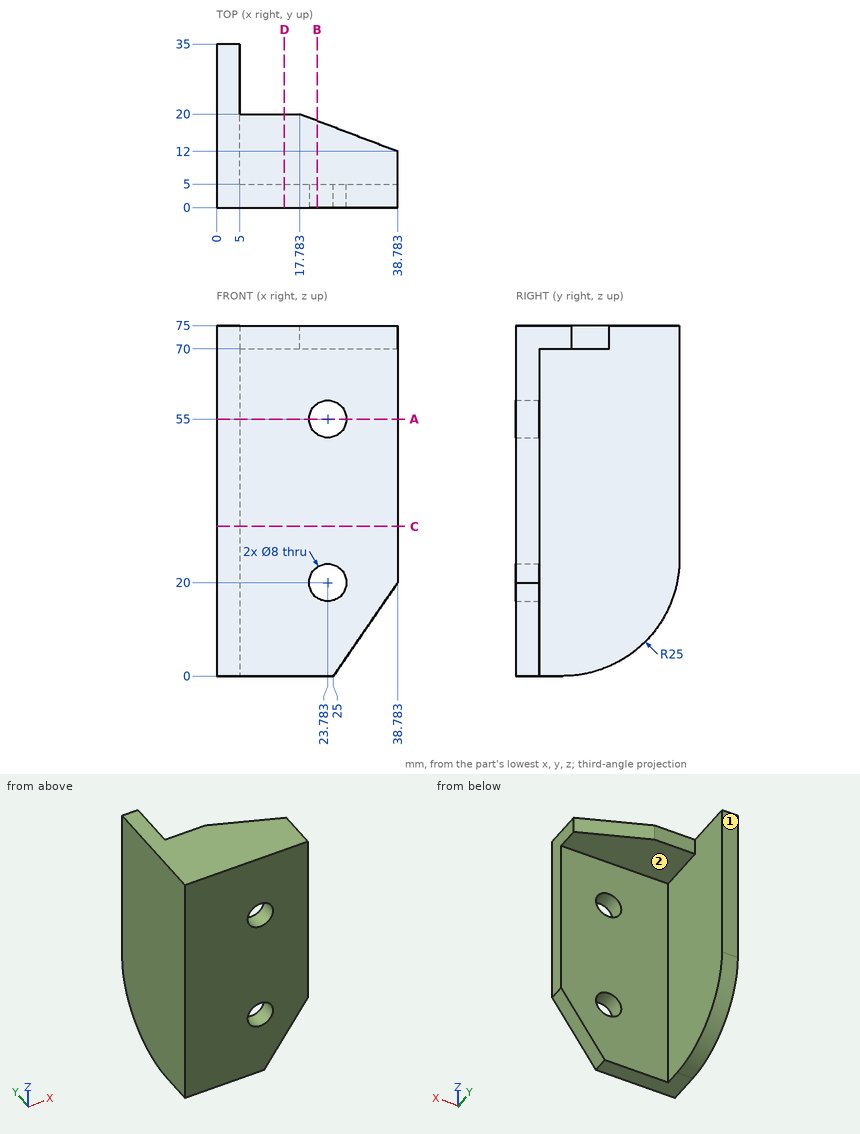
The drawing under review shows one solid part. Ordinate dimensions are in mm from its lowest x, y, z. A direction names the side the tool comes from. Round coordinates to 2 decimals unless told otherwise and drop trailing zeros. Loops run counter-clockwise (first coordinate to the right, second up) from the corner with the lowest first, then second, coordinate; pieces in that order, holes last. Notation, with made-up numbers: (-19, 12.25) - (27, 12.25) arc R7 ccw to (27, 18.25) - close; hole circle Ø2 at (0, -22). An arc over 180 degrees is marked (long way). One line per question, with ' | ' between items.
1. For L1, parallel to Y at x = 13.5, z = 48; L2, parallel to Z at x = 18.5, y = 11, list the stretches that pass through material, from the lowest coordinate up. Write a range as [from, to].
Results are:
L1: y = [0, 5] | L2: z = [70, 75]
2. For the marked faces 1 and 2, list the 3-axis set-ups (+Z, -Z, +X, -X, +Y, -Y) from which the entire face can be reached by the end or side of a thin tool; tool diameter is ignored.
Results are:
face 1: +Z, -Z, +X, -X, +Y | face 2: -Z, +X, +Y
3. Clearance check with flat-ended pins moving along their axes: P1, Ø1, axis at y = 22.5, z = 17, coming from the -X side; P2, Ø6.5, axis at x = 23.78, z = 20, coming from the -Y side (1 decimal); P3, Ø3, axis at y = 11.5, z = 26, coming from the +X side; P4, Ø5.5, axis at x = 11.5, z = 72.5, coming from the +Y side. State where each tip first meets the part, or that it passes through.
Results are:
P1: stops at x = 0 | P2: passes through | P3: stops at x = 5 | P4: stops at y = 20
4. We need section B-B, the plane x = 21.5. State the section outline as (y, z) points.
Results are:
outline: (0, 0) - (5, 0) - (5, 16.72) - (0, 16.72) - close; (0, 23.28) - (5, 23.28) - (5, 51.72) - (0, 51.72) - close; (0, 58.28) - (5, 58.28) - (5, 70) - (18.58, 70) - (18.58, 75) - (0, 75) - close
5. We need section A-A, the plane z = 55. State the section outline as (x, y) points, and give its area (3 significant figures).
Results are:
outline: (0, 0) - (19.78, 0) - (19.78, 5) - (5, 5) - (5, 35) - (0, 35) - close; (27.78, 0) - (38.78, 0) - (38.78, 5) - (27.78, 5) - close | area: 304 mm²
6. We need section D-D, the plane x = 14.5. State the section outline as (y, z) points, and give its area (3 significant figures).
Results are:
outline: (0, 0) - (5, 0) - (5, 70) - (20, 70) - (20, 75) - (0, 75) - close | area: 450 mm²
7. We need section C-C, the plane z = 32. State the section outline as (x, y) points, and give its area (3 significant figures).
Results are:
outline: (0, 0) - (38.78, 0) - (38.78, 5) - (5, 5) - (5, 35) - (0, 35) - close | area: 344 mm²
